Check sheet for the modelled part. Datum: model origin and axes. Units: mm. Face numbers are marked on the shaded views. A direction names the side the tool comes from. Give positions to 0.01 mm unless a question says otherwise; leave off trailing zeros. Write each loop counter-clockwise with the first axis right and the second up, starting at its lowest first coordinate (ties: lowest second). Pieces come first, ordered by that corner, then holes. Notation, with made-up numbers: M 34,8.5 L 64,8.5 A26 cw 64,35.5 Z; hole C 43.5,27.5 d10. An arc over 180 degrees is marked long. Use CSV: the item, a comma, the result in double quotes. Start each with the question number.
1. Cross-section at C-C, the plane z = 6.25. Enter the section's corners in (x, y), and give its area (3 significant figures).
2. Cross-section at D-D, the plane x = -5.5. Enter the section's corners in (y, z).
3. Cross-section at A-A, the plane x = 0. Enter the section's corners in (y, z), and give its area (3 significant figures).
4. Depth check by flat-ended pin: P1, Ø2, axis at y = 5.5, z = 3.5, coming from the -X side; P2, Ø3, axis at x = 0.5, y = -2.5, coming from the -Z side; P3, Ø2, axis at x = 1.5, z = 1, coming from the -Y side. Enter the tip coordinate at first touch or a pass-through.
5. Mould release check, pull along X, two halves, no side actions. Record for the marked faces 4, 5 and 6: +X half, -X half, draft (parallel to the pull), parting line (faces both ways), or undercut.
6. Access from +Z, -Z, +X, -X, +Y, -Y to the whole of each face (thin tool, end or side, straight path). Record for the marked faces 1, 2 and 3.
7. Scan lines: line 1 (Y direction, x = 0, z = 0.6); line 2 (Y direction, x = 0, z = 6.1); line 3 (X direction, y = 0, z = 4.6). Record each from-to range of solid material in increasing order.
from build123d import *


with BuildPart() as part:
    # Sketch2 → Revolve1 (revolve)
    with BuildSketch(Plane(origin=(0, 0, 0), x_dir=(1, 0, 0), z_dir=(0, 1, 0))):
        Polygon((-3.5, -6.7), (-3.5, -5.9), (-4.8, -5.58), (-4.8, -3.08), (-3.3, -3.08), (-3.3, -1), (-5, -1), (-5, -0.4), (-5.3, -0.4), (-5.3, 0), (-7, 0), (-7, -0.2), (-6.8, -0.2), (-6.8, -6.7), align=None)
    revolve(axis=Axis((0, 0, 0), (0, 0, 1)))


solid = part.part
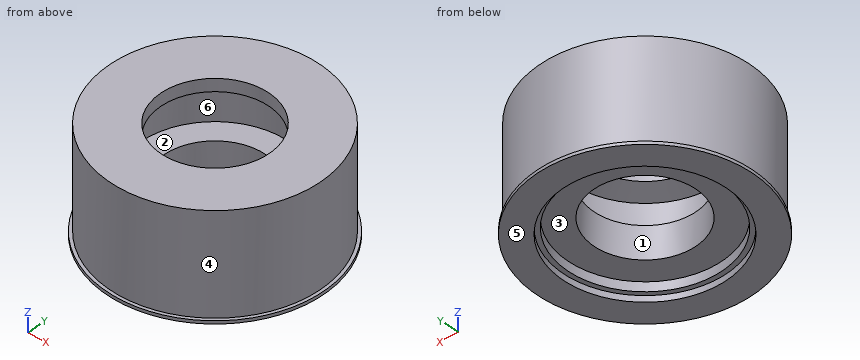
Worked answers:
1,outline,"C 0,0 d13.6; hole C 0,0 d7"
1,area,"107 mm^2"
2,outline,"M -4.33,0 L 4.33,0 L 4.33,0.2 L 4,0.2 L 4,6.7 L -4,6.7 L -4,0.2 L -4.33,0.2 Z"
3,outline,"M -7,0 L -5.3,0 L -5.3,0.4 L -5,0.4 L -5,1 L -3.3,1 L -3.3,3.08 L -4.8,3.08 L -4.8,5.58 L -3.5,5.9 L -3.5,6.7 L -6.8,6.7 L -6.8,0.2 L -7,0.2 Z; M 3.3,1 L 5,1 L 5,0.4 L 5.3,0.4 L 5.3,0 L 7,0 L 7,0.2 L 6.8,0.2 L 6.8,6.7 L 3.5,6.7 L 3.5,5.9 L 4.8,5.58 L 4.8,3.08 L 3.3,3.08 Z"
3,area,"35.0 mm^2"
4,P1,"stops at x = -5.1"
4,P2,"stops at z = 1"
4,P3,"stops at y = -6.94"
5,face 4,"parting line"
5,face 5,"draft"
5,face 6,"undercut"
6,face 1,"+Z, -Z"
6,face 2,"none"
6,face 3,"-Z"
7,line 1,"y = -6.8 to -5, 5 to 6.8"
7,line 2,"y = -6.8 to -3.5, 3.5 to 6.8"
7,line 3,"x = -6.8 to -4.8, 4.8 to 6.8"
